Work out the finished part from the listing and answer in its coordinate system (mm). Give positions to 0.01 mm unless a question says otherwise; leave off trailing zeros. Order: outer loops, then holes, each group sorted by start corner. A loop starts at its lowest first (then second) coordinate and runs counter-clockwise, first axis right, second up.
```python
from build123d import *

# Parameters (mm, degrees)
SKETCH1_R           = 2
BOSS_EXTRUDE1_DEPTH = 5
BOSS_EXTRUDE2_DEPTH = 5
SKETCH3_R           = 1.25
CUT_EXTRUDE1_DEPTH  = 5


with BuildPart() as part:
    # Sketch1 → Boss-Extrude1 (new body)
    with BuildSketch(Plane.XY):
        with BuildLine():
            Line((-60, -85), (-26.662742925, -85))
            ThreePointArc((-26.662742925, -85), (-25.208437327, -85.376072556), (-24.118748013, -86.41000318))
            Line((-24.118748013, -86.41000318), (-20.881251987, -91.58999682))
            ThreePointArc((-20.881251987, -91.58999682), (-19.791562673, -92.623927444), (-18.337257075, -93))
            Line((-18.337257075, -93), (18.337257075, -93))
            ThreePointArc((18.337257075, -93), (19.791562673, -92.623927444), (20.881251987, -91.58999682))
            Line((20.881251987, -91.58999682), (24.118748013, -86.41000318))
            ThreePointArc((24.118748013, -86.41000318), (25.208437327, -85.376072556), (26.662742925, -85))
            Line((26.662742925, -85), (60, -85))
            ThreePointArc((60, -85), (63.535533906, -83.535533906), (65, -80))
            Line((65, -80), (65, 80))
            ThreePointArc((65, 80), (63.535533906, 83.535533906), (60, 85))
            Line((60, 85), (26.662742925, 85))
            ThreePointArc((26.662742925, 85), (25.208437327, 85.376072556), (24.118748013, 86.41000318))
            Line((24.118748013, 86.41000318), (20.881251987, 91.58999682))
            ThreePointArc((20.881251987, 91.58999682), (19.791562673, 92.623927444), (18.337257075, 93))
            Line((18.337257075, 93), (-18.337257075, 93))
            ThreePointArc((-18.337257075, 93), (-19.791562673, 92.623927444), (-20.881251987, 91.58999682))
            Line((-20.881251987, 91.58999682), (-24.118748013, 86.41000318))
            ThreePointArc((-24.118748013, 86.41000318), (-25.208437327, 85.376072556), (-26.662742925, 85))
            Line((-26.662742925, 85), (-60, 85))
            ThreePointArc((-60, 85), (-63.535533906, 83.535533906), (-65, 80))
            Line((-65, 80), (-65, -80))
            ThreePointArc((-65, -80), (-63.535533906, -83.535533906), (-60, -85))
        make_face()
        with Locations((-10, 89)):
            Circle(SKETCH1_R, mode=Mode.SUBTRACT)
        with Locations((10, 89)):
            Circle(SKETCH1_R, mode=Mode.SUBTRACT)
        with Locations((10, -89)):
            Circle(SKETCH1_R, mode=Mode.SUBTRACT)
        with Locations((-10, -89)):
            Circle(SKETCH1_R, mode=Mode.SUBTRACT)
    extrude(amount=BOSS_EXTRUDE1_DEPTH)

    # Sketch2 → Boss-Extrude2 (add)
    with BuildSketch(Plane.XY.offset(5)):
        with BuildLine():
            Line((60, -85), (-60, -85))
            ThreePointArc((-60, -85), (-63.535533906, -83.535533906), (-65, -80))
            Line((-65, -80), (-65, 80))
            ThreePointArc((-65, 80), (-63.535533906, 83.535533906), (-60, 85))
            Line((-60, 85), (60, 85))
            ThreePointArc((60, 85), (63.535533906, 83.535533906), (65, 80))
            Line((65, 80), (65, -80))
            ThreePointArc((65, -80), (63.535533906, -83.535533906), (60, -85))
        make_face()
    extrude(amount=BOSS_EXTRUDE2_DEPTH)

    # Sketch3 → Cut-Extrude1 (cut)
    with BuildSketch(Plane.XY.offset(10)):
        with Locations((60, -27)):
            Circle(SKETCH3_R)
        with Locations((60, -80)):
            Circle(SKETCH3_R)
        with Locations((-60, -27)):
            Circle(SKETCH3_R)
        with Locations((-60, -80)):
            Circle(SKETCH3_R)
        with Locations((0, -80)):
            Circle(SKETCH3_R)
        with Locations((60, 27)):
            Circle(SKETCH3_R)
        with Locations((60, 80)):
            Circle(SKETCH3_R)
        with Locations((0, 80)):
            Circle(SKETCH3_R)
        with Locations((-60, 27)):
            Circle(SKETCH3_R)
        with Locations((-60, 80)):
            Circle(SKETCH3_R)
        with Locations((-20, -67)):
            Circle(SKETCH3_R)
        with Locations((-20, -44)):
            Circle(SKETCH3_R)
        with Locations((-20, -22)):
            Circle(SKETCH3_R)
        with Locations((-20, 0)):
            Circle(SKETCH3_R)
        with Locations((-20, 22)):
            Circle(SKETCH3_R)
        with Locations((-20, 44)):
            Circle(SKETCH3_R)
        with Locations((-20, 67)):
            Circle(SKETCH3_R)
        with Locations((36, -52)):
            Circle(SKETCH3_R)
        with Locations((36, -36)):
            Circle(SKETCH3_R)
        with Locations((36, 8)):
            Circle(SKETCH3_R)
        with Locations((36, -8)):
            Circle(SKETCH3_R)
        with Locations((36, 52)):
            Circle(SKETCH3_R)
        with Locations((36, 36)):
            Circle(SKETCH3_R)
        with Locations((20, -67)):
            Circle(SKETCH3_R)
        with Locations((20, -22)):
            Circle(SKETCH3_R)
        with Locations((20, 22)):
            Circle(SKETCH3_R)
        with Locations((20, 67)):
            Circle(SKETCH3_R)
        with Locations((12, -44)):
            Circle(SKETCH3_R)
        with Locations((12, 0)):
            Circle(SKETCH3_R)
        with Locations((12, 44)):
            Circle(SKETCH3_R)
    extrude(amount=-CUT_EXTRUDE1_DEPTH, mode=Mode.SUBTRACT)


solid = part.part
```
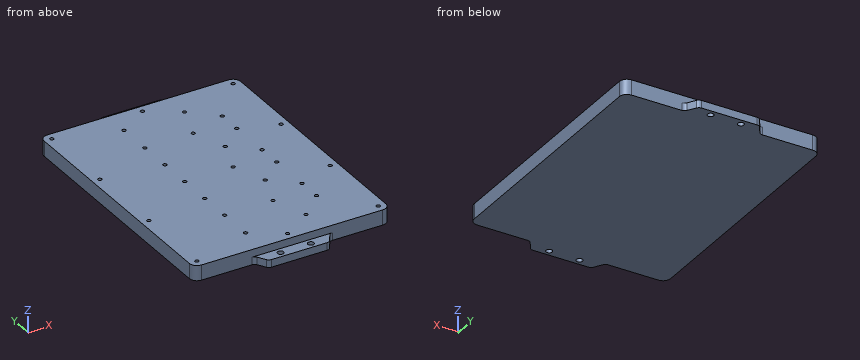
1. The part is cut by section A-A (x = -10). Write down the section's boundary in (y, z).
Findings below:
outline: (-93, 0) - (-91, 0) - (-91, 5) - (-93, 5) - close; (-87, 0) - (87, 0) - (87, 5) - (85, 5) - (85, 10) - (-85, 10) - (-85, 5) - (-87, 5) - close; (91, 0) - (93, 0) - (93, 5) - (91, 5) - close
2. Given P1, Ø6, axis at x = 49.5, z = 5, coming from the +Y side; P2, Ø2, axis at x = -60, y = -80, coming from the +Z side, each flat-ended and moving along its own axis, determine where each tip first touches the part or whether it passes through.
Findings below:
P1: stops at y = 85
P2: stops at z = 5
3. The part is cut by section C-C (x = 45). Write down the section's boundary in (y, z).
Findings below:
outline: (-85, 0) - (85, 0) - (85, 10) - (-85, 10) - close
4. Straight lines are drawn through the part: probe 1 along Y at (x, z) = (12, 8.4); probe 2 along Y at (x, z) = (60, 8.25); probe 3 along Y at (x, z) = (-36.5, 9.5). For each, find the intervals that lie inside material, in ascending order.
Findings below:
probe 1: y = -85 to -45.25, -42.75 to -1.25, 1.25 to 42.75, 45.25 to 85
probe 2: y = -85 to -81.25, -78.75 to -28.25, -25.75 to 25.75, 28.25 to 78.75, 81.25 to 85
probe 3: y = -85 to 85
5. The part is cut by section B-B (z = 3.5). Write down the section's boundary in (x, y), then the cut area to 3 significant figures.
Findings below:
outline: (-65, -80) arc R5 ccw to (-60, -85) - (-26.66, -85) arc R3 cw to (-24.12, -86.41) - (-20.88, -91.59) arc R3 ccw to (-18.34, -93) - (18.34, -93) arc R3 ccw to (20.88, -91.59) - (24.12, -86.41) arc R3 cw to (26.66, -85) - (60, -85) arc R5 ccw to (65, -80) - (65, 80) arc R5 ccw to (60, 85) - (26.66, 85) arc R3 cw to (24.12, 86.41) - (20.88, 91.59) arc R3 ccw to (18.34, 93) - (-18.34, 93) arc R3 ccw to (-20.88, 91.59) - (-24.12, 86.41) arc R3 cw to (-26.66, 85) - (-60, 85) arc R5 ccw to (-65, 80) - close; hole circle Ø4 at (-10, -89); hole circle Ø4 at (-10, 89); hole circle Ø4 at (10, -89); hole circle Ø4 at (10, 89)
area: 22,700 mm2
